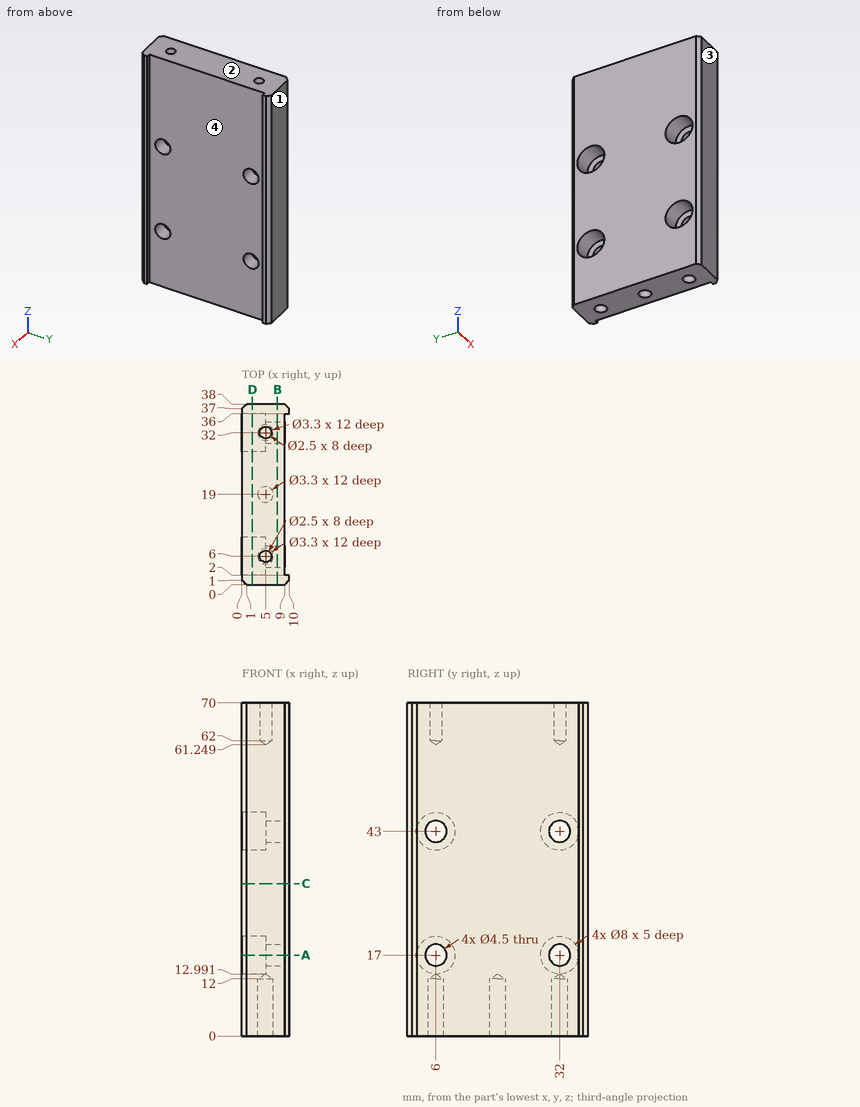
Job drawing, mm, ordinate dimensions from the low corner. One solid piece. Round coordinates to 2 decimals unless told otherwise and drop trailing zeros. Loops run counter-clockwise (first coordinate to the right, second up) from the corner with the lowest first, then second, coordinate; pieces in that order, holes last. Notation, with made-up numbers: (47, 77) -> (72, 77) arc R24 ccw to (72, 91) -> close; hole circle Ø5 at (-1, -32.5). An arc over 180 degrees is marked (long way). One line per item, written item: value. Start each with the question number.
Q1. Drop flat-ended pins along their axis: pin 1 Ø1.5 at (x, z) = (2, 22) entering from -Y; pin 2 Ø6.5 at (y, z) = (6, 17) entering from -X; pin 3 Ø10 at (y, z) = (26, 51.5) entering from +X; pin 4 Ø2 at (x, y) = (5, 32) entering from +Z. Give the stop position or say it passes through.
Q2. Probe line 1 along Z through (x, y) = (6.8, 32); line 2 along Z through (x, y) = (1.25, 6); line 3 along Y through (x, z) = (5, 8). List the from-to ranges inside material, lowest first.
Q3. Two-plate mould, pull along Y, no slides. Class the marked faces 1, 2, 3 and 4: released by +Y, released by -Y, zero draft, split by the parting line, or undercut.
Q4. Cut at D-D on x = 2.25. List the corners of the cut face in (y, z).
Q5. Cut at C-C on z = 32. List the corners of the cut face in (x, y), plus the area to 3 significant figures.
Q6. Cut at A-A on z = 17. List the corners of the cut face in (x, y).
Q7. Cut at B-B on x = 7.5. List the corners of the cut face in (y, z).
Computed:
1. pin 1: y = 0
1. pin 2: x = 5
1. pin 3: x = 9
1. pin 4: z = 61.85
2. line 1: 0 to 14.75, 19.25 to 40.75, 45.25 to 70
2. line 2: 0 to 13, 21 to 39, 47 to 70
2. line 3: 0 to 4.35, 7.65 to 17.35, 20.65 to 30.35, 33.65 to 38
3. face 1: released by +Y
3. face 2: zero draft
3. face 3: released by -Y
3. face 4: undercut
4. outline: (0, 0) -> (38, 0) -> (38, 70) -> (0, 70) -> close; hole circle Ø8 at (6, 17); hole circle Ø8 at (6, 43); hole circle Ø8 at (32, 17); hole circle Ø8 at (32, 43)
5. outline: (0, 1) -> (1, 0) -> (9, 0) -> (10, 1) -> (10, 2) -> (9, 2) -> (9, 36) -> (10, 36) -> (10, 37) -> (9, 38) -> (1, 38) -> (0, 37) -> close
5. area: 344 mm²
6. outline: (0, 1) -> (1, 0) -> (9, 0) -> (10, 1) -> (10, 2) -> (9, 2) -> (9, 3.75) -> (5, 3.75) -> (5, 2) -> (0, 2) -> close; (0, 10) -> (5, 10) -> (5, 8.25) -> (9, 8.25) -> (9, 29.75) -> (5, 29.75) -> (5, 28) -> (0, 28) -> close; (0, 36) -> (5, 36) -> (5, 34.25) -> (9, 34.25) -> (9, 36) -> (10, 36) -> (10, 37) -> (9, 38) -> (1, 38) -> (0, 37) -> close
7. outline: (0, 0) -> (38, 0) -> (38, 70) -> (0, 70) -> close; hole circle Ø4.5 at (6, 17); hole circle Ø4.5 at (6, 43); hole circle Ø4.5 at (32, 17); hole circle Ø4.5 at (32, 43)
